Can you work these out from the drawing? Everything is in mm from the part's minimum corner. A direction names the side the tool comes from. Round coordinates to 2 decimals unless told otherwise and drop trailing zeros. Write each loop counter-clockwise with the first axis right and the second up, starting at its lowest first coordinate (ties: lowest second). Pieces come first, ordered by that corner, then holes. Notation, with made-up numbers: (85.25, 65) -> (102.25, 65) arc R10 ccw to (102.25, 81) -> close; hole circle Ø2 at (13.25, -4). An arc over 180 degrees is marked (long way). One line per question, with ' | ' between items. Start each with the question number.
1. For pin 1 Ø2 at (y, z) = (4.5, 69) entering from -X; pin 2 Ø3 at (y, z) = (1, 66) entering from -X; pin 3 Ø1.6 at (y, z) = (5, 4.5) entering from +X; pin 4 Ø1.2 at (x, y) = (19, 2.5) entering from -Z, each with a flat end and sliding along its axis, tell me the tip position at first contact or that it passes through.
2. If I drill on line 1 along Z through (x, y) = (14.5, 5.3); line 2 along Y through (x, z) = (18, 71); line 3 along Z through (x, y) = (19, 3.5), over which ranges is the centre line in solid material (lowest first)? Write a range as [from, to].
3. Imagine slicing it at B-B, the plane z = 15. List the corners of the cut face in (x, y) for me.
4. Imagine slicing it at A-A, the plane x = 15. List the corners of the cut face in (y, z) for me, and give its area (3 significant figures).
5. For the marked faces 1 and 2, which set-ups out of +Z, -Z, +X, -X, +Y, -Y let a thin tool reach every point of the face, with its end or its side?
6. Imagine slicing it at C-C, the plane y = 1.05. List the corners of the cut face in (x, z) for me.
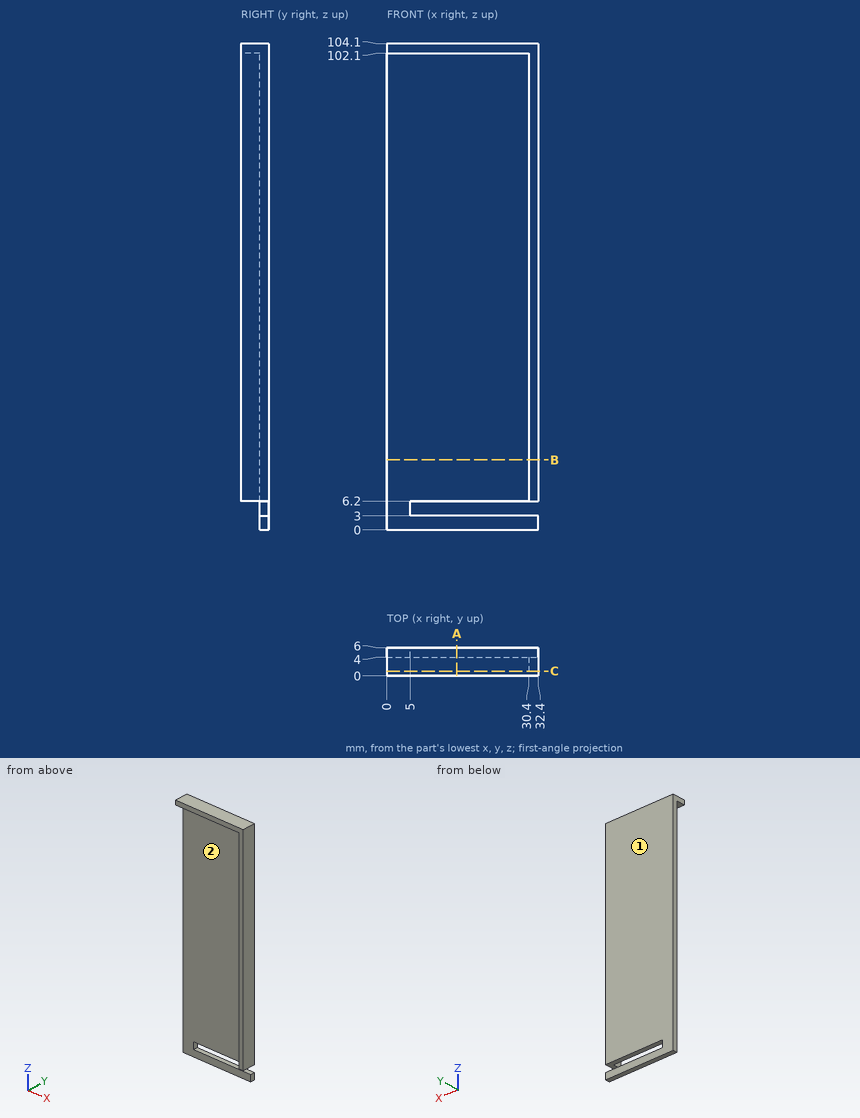
Geometry results:
1) pin 1: stops at x = 0 | pin 2: stops at x = 30.4 | pin 3: stops at x = 5 | pin 4: stops at z = 102.1
2) line 1: z = [0, 3], [6.2, 104.1] | line 2: y = [4, 6] | line 3: z = [102.1, 104.1]
3) outline: (0, 4) -> (30.4, 4) -> (30.4, 0) -> (32.4, 0) -> (32.4, 6) -> (0, 6) -> close
4) outline: (0, 102.1) -> (4, 102.1) -> (4, 6.2) -> (6, 6.2) -> (6, 104.1) -> (0, 104.1) -> close; (4, 0) -> (6, 0) -> (6, 3) -> (4, 3) -> close | area: 210 mm2
5) face 1: +Z, -Z, +X, -X, +Y | face 2: -Z, -X, -Y
6) outline: (0, 102.1) -> (30.4, 102.1) -> (30.4, 6.2) -> (32.4, 6.2) -> (32.4, 104.1) -> (0, 104.1) -> close
